from build123d import *

# Parameters (mm, degrees)
SKETCH3_W             = 2
SKETCH3_H             = 5
BOSS_EXTRUDE1_DEPTH   = 30
BOSS_EXTRUDE1_2_DEPTH = 30
SKETCH4_W             = 5
SKETCH4_H             = 5
CUT_EXTRUDE1_DEPTH    = 1
SKETCH5_W             = 5
SKETCH5_H             = 5
CUT_EXTRUDE2_DEPTH    = 1
SWEEP1_START          = 8
SWEEP1_DEPTH          = 14
SKETCH7_R             = 1.5
BOSS_EXTRUDE2_DEPTH   = 1
BOSS_EXTRUDE3_START   = 1
SKETCH8_R             = 1.5
BOSS_EXTRUDE3_DEPTH   = 1
FILLET1_R             = 2.5
CUT_EXTRUDE3_DEPTH    = 1
CUT_EXTRUDE4_DEPTH    = 1
FILLET2_R             = 2.5


# Read off the part's stored shape, not the designer's step: Sweep1
with BuildPart() as part:
    # Sketch3 → Boss-Extrude1 (new body)
    with BuildSketch(Plane(origin=(0, 0, 0), x_dir=(0, 0, -1), z_dir=(1, 0, 0))):
        with Locations((-10, 0)):
            Rectangle(SKETCH3_W, SKETCH3_H)
    extrude(amount=BOSS_EXTRUDE1_DEPTH)

    # Sketch4 → Cut-Extrude1 (cut)
    with BuildSketch(Plane.XY.offset(11)):
        with Locations((2.5, 0)):
            Rectangle(SKETCH4_W, SKETCH4_H)
        with Locations((27.5, 0)):
            Rectangle(SKETCH4_W, SKETCH4_H)
    extrude(amount=-CUT_EXTRUDE1_DEPTH, mode=Mode.SUBTRACT)



with BuildPart() as body_2:
    # Sketch3 → Boss-Extrude1 2 (new body)
    with BuildSketch(Plane(origin=(0, 0, 0), x_dir=(0, 0, -1), z_dir=(1, 0, 0))):
        with Locations((10, 0)):
            Rectangle(SKETCH3_W, SKETCH3_H)
    extrude(amount=BOSS_EXTRUDE1_2_DEPTH)

    # Sketch5 → Cut-Extrude2 (cut)
    with BuildSketch(Plane(origin=(0, 0, -11), x_dir=(-1, 0, 0), z_dir=(0, 0, -1))):
        with Locations((-27.5, 0)):
            Rectangle(SKETCH5_W, SKETCH5_H)
        with Locations((-2.5, 0)):
            Rectangle(SKETCH5_W, SKETCH5_H)
    extrude(amount=-CUT_EXTRUDE2_DEPTH, mode=Mode.SUBTRACT)


with BuildPart() as part_1:
    add(part.part)

    add(body_2.part)  # Sweep1 merges body 2
    # Sweep1 outline → Sweep1 (add)
    with BuildSketch(Plane.YZ.offset(SWEEP1_START)):
        with BuildLine():
            Line((2.5, -9), (2.5, -11))
            ThreePointArc((2.5, -11), (13.5, 0), (2.5, 11))
            Line((2.5, 11), (2.5, 9))
            ThreePointArc((2.5, 9), (11.5, 0), (2.5, -9))
        make_face()
    extrude(amount=SWEEP1_DEPTH)

    # Sketch7 → Boss-Extrude2 (add)
    with BuildSketch(Plane(origin=(0, 0, -10), x_dir=(-1, 0, 0), z_dir=(0, 0, -1))):
        with Locations(Location((-2.5, 0, 0), (0, 0, 270))):
            Circle(SKETCH7_R)
        with Locations(Location((-27.5, 0, 0), (0, 0, 90))):
            Circle(SKETCH7_R)
    extrude(amount=BOSS_EXTRUDE2_DEPTH)

    # Sketch8 → Boss-Extrude3 (add)
    with BuildSketch(Plane.XY.offset(10).offset(BOSS_EXTRUDE3_START)):
        with Locations(Location((27.5, 0, 0), (0, 0, 90))):
            Circle(SKETCH8_R)
        with Locations(Location((2.5, 0, 0), (0, 0, 270))):
            Circle(SKETCH8_R)
    extrude(amount=-BOSS_EXTRUDE3_DEPTH)

    # Fillet1
    fillet1_edges = [part_1.edges().sort_by_distance(p)[0] for p in [
        (0, -2.5, 9.5),
        (30, -2.5, 9.5),
        (30, -2.5, -9.5),
        (0, -2.5, -9.5),
    ]]
    fillet(fillet1_edges, radius=FILLET1_R)

    # Sketch9 → Cut-Extrude3 (cut)
    with BuildSketch(Plane.XY.offset(11)):
        Polygon((5, 2.5), (7.5, -2.5), (5, -2.5), align=None)
    extrude(amount=-CUT_EXTRUDE3_DEPTH, mode=Mode.SUBTRACT)

    # Sketch10 → Cut-Extrude4 (cut)
    with BuildSketch(Plane(origin=(0, 0, -11), x_dir=(-1, 0, 0), z_dir=(0, 0, -1))):
        Polygon((-5, 2.5), (-7.5, -2.5), (-5, -2.5), align=None)
    extrude(amount=-CUT_EXTRUDE4_DEPTH, mode=Mode.SUBTRACT)

    # Fillet2
    fillet2_edges = [part_1.edges().sort_by_distance(p)[0] for p in [
        (25, -2.5, 10.5),
        (25, -2.5, -10.5),
    ]]
    fillet(fillet2_edges, radius=FILLET2_R)


solid = part_1.part
Here's how the part is built. I have some questions about the finished solid (model axes, mm). A direction names the side the tool comes from. Coordinates: 2 decimals unless noted, no trailing zeros. Loops run counter-clockwise (first coordinate to the right, second up) from the corner with the lowest first, then second, coordinate; pieces in that order, holes last.
1. Imagine slicing it at B-B, the plane y = 8. Please give me the cut outline in (x, z), and give its area (3 significant figures).
2. For faces 1 (the flat face through (25.1, 2.5, -9.8)), 2 (the flat face through (25, 1.2, -10.5)), 3 (the flat face through (4.8, 2.5, -9.8)), 4 (the flat face through (15, 0, -9)), 5 (the cylindrical face through (1.036, 0.325, 10.507)), which set-ups out of +Z, -Z, +X, -X, +Y, -Y let a thin tool reach every point of the face, with its end or its side?
3. I need wall thicknesses on L1, parallel to Z at x = 11.5, y = 1; L2, parallel to Z at x = 18.25, y = 7.5; L3, parallel to X at y = 6, z = -9.5. Which ranges of each line are inside material? Lowest first, please.
4. Imagine slicing it at A-A, the plane x = 6.75. Please give me the cut outline in (y, z), and give its area (3 significant figures).
5. If we mould it in two halves opening along X, with no side actions, what happens to faces 6 (the flat face through (30, 1.3, 9.5)), 7 (the flat face through (27, 0, 11)), 8 (the flat face through (25, 1.2, 10.5))? For each: pulls with the +X half, pulls with the -X half, needs draft (parallel to the pull), parting line crosses it, or undercut.
6. Imagine slicing it at C-C, the plane x = 11.25. Please give me the cut outline in (y, z).
7. For P1, Ø0.5, axis at y = 0.5, z = 10.5, coming from the +X side; P2, Ø2, axis at x = 5, z = 10, coming from the +Y side; P3, Ø10, axis at x = 5.5, z = 7.5, coming from the +Y side, each with a flat end and sliding along its axis, tell me the tip position at first contact or that it passes through.
8. Imagine slicing it at D-D, the plane z = 0. Please give me the cut outline in (x, y).
Taken from the geometry:
1. outline: (8, -9.53) - (22, -9.53) - (22, -7.12) - (8, -7.12) - close; (8, 7.12) - (22, 7.12) - (22, 9.53) - (8, 9.53) - close
1. area: 67.3 mm2
2. face 1: +Z, -Z, +X, +Y
2. face 2: -Z, +Y, -Y
2. face 3: +Z, -Z, -X, +Y
2. face 4: +X, -X, -Y
2. face 5: +Z
3. L1: z = -11 to -9, 9 to 11
3. L2: z = -9.8 to -7.48, 7.48 to 9.8
3. L3: x = 8 to 22
4. outline: (-2.5, -10) - (-1, -10) - (-1, -11) - (2.5, -11) - (2.5, -9) - (-2.5, -9) - close; (-2.5, 9) - (2.5, 9) - (2.5, 11) - (-1, 11) - (-1, 10) - (-2.5, 10) - close
4. area: 17.0 mm2
5. face 6: pulls with the +X half
5. face 7: needs draft
5. face 8: undercut
6. outline: (-2.5, -11) - (2.5, -11) arc R11 ccw to (2.5, 11) - (-2.5, 11) - (-2.5, 9) - (2.5, 9) arc R9 cw to (2.5, -9) - (-2.5, -9) - close
7. P1: stops at x = 28.98
7. P2: stops at y = 2.5
7. P3: stops at y = 13.03
8. outline: (8, 11.5) - (22, 11.5) - (22, 13.5) - (8, 13.5) - close
